Verification items for the finished model (mm, model axes). Face numbers are marked on the shaded views. A direction names the side the tool comes from. Coordinates: 2 decimals unless noted, no trailing zeros. Loops run counter-clockwise (first coordinate to the right, second up) from the corner with the lowest first, then second, coordinate; pieces in that order, holes last. Notation, with made-up numbers: (-6.5, -22.75) -> (23.5, -22.75) arc R5 ccw to (23.5, -17.75) -> close; hole circle Ø4 at (23, 5). An arc over 180 degrees is marked (long way). Answer as a JSON object with one key per item and string values. Group by question number.
Q1. Cross-section at A-A on x = 930.5. Record the boundary of the cut face in (y, z).
Q2. Cross-section at C-C on z = 60.5. Record the boundary of the cut face in (x, y).
Q3. Scan lines: L1, parallel to Z at x = 25, y = 391.1; L2, parallel to Z at x = 851, y = 26; L3, parallel to Y at x = 1153, z = 30. Record each from-to range of solid material in increasing order.
Q4. Set-up check for the marked faces 1, 2 and 3: record each of +Z, -Z, +X, -X, +Y, -Y from which the full face is reachable in a straight line by a thin tool's end or side.
Q5. Gauge pin test, flat ends, axial feed: pin 1 Ø4 at (x, z) = (692, 48) entering from -Y; pin 2 Ø4 at (x, y) = (1523, 350) entering from +Z; pin 3 Ø15.5 at (x, z) = (545, 204.8) entering from +Y; pin 4 Ø11 at (x, z) = (25, 174.8) entering from +Y. Record the tip position at first contact, or that the pin passes through.
Q6. Cross-section at B-B on y = 361.5. Record the boundary of the cut face in (x, z).
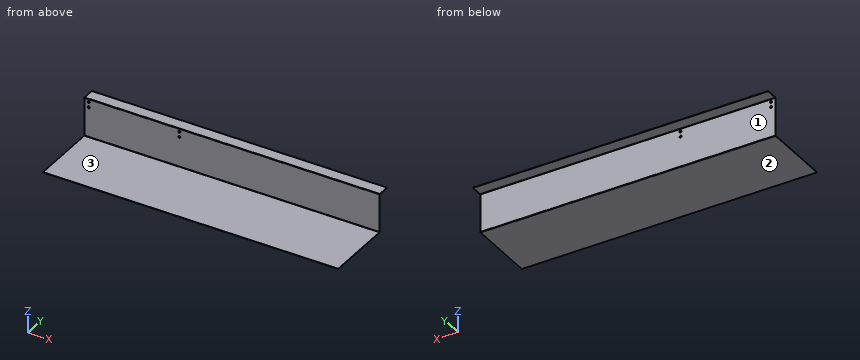
Autodesk Inventor part; units mm, degrees
ref_plane "YZ Plane" through (0, 0, 0) normal (1, 0, 0) x (0, 1, 0)
ref_plane "XZ Plane" through (0, 0, 0) normal (0, 1, 0) x (-1, 0, 0)
ref_plane "XY Plane" through (0, 0, 0) normal (0, 0, 1) x (1, 0, 0)
sketch "Sketch1" plane through (0, 0, 0) normal (0, 0, 1) x (1, 0, 0)
  line L0 (0, 0) -> (0, 392)
  line L1 (0, 392) -> (1695, 392)
  line L2 (1695, 392) -> (1695, 0)
  line L3 (1695, 0) -> (0, 0)
  dimension "d0" = 392
  dimension "d1" = 1695
extrude "Plate1" add sketch "Sketch1" along normal blind 1.6
sketch "Sketch2" plane through (1695, 390.4, 0) normal (0, 1, 0) x (-1, 0, 0)
  line L0 (1695, 0) -> (0, 0)
  line L1 (0, 0) -> (0, -223)
  line L2 (0, -223) -> (1695, -223)
  line L3 (1695, -223) -> (1695, 0)
edge flange "Flange1" height 223 angle 90 thickness 1.6 bend radius 1.6 thickness toward (0, 1, 0) relief tear relief width 1.6 relief depth 0.8 edges at (847.5, 392, 0) wall of the first edge with corners at (0, 390.4, 0) (1695, 390.4, 0) (1695, 390.4, 223) (0, 390.4, 223)
bend "Bend1"
corner "Corner1"
sketch "Sketch3" plane through (0, 390.4, 221.4) normal (0, 0, 1) x (1, 0, 0)
  line L0 (1695, 0) -> (0, 0)
  line L1 (0, 0) -> (0, -70)
  line L2 (0, -70) -> (1695, -70)
  line L3 (1695, -70) -> (1695, 0)
edge flange "Flange2" height 70 angle -90 thickness 1.6 bend radius 1.6 thickness toward (0, 0, 1) relief tear relief width 1.6 relief depth 0.8 edges at (847.5, 390.4, 223) wall of the first edge with corners at (1695, 390.4, 221.4) (0, 390.4, 221.4) (0, 460.4, 221.4) (1695, 460.4, 221.4)
bend "Bend2"
corner "Corner2"
sketch "Sketch4" plane through (0, 390.4, 3.2) normal (0, -1, 0) x (1, 0, 0)
  line L0 (0, 0) -> (0, 216.6)
  line L1 (0, 216.6) -> (0, 156.6)
  line L2 (0, 156.6) -> (1695, 156.6)
  line L3 (1695, 216.6) -> (1695, 0)
  line L4 (1695, 216.6) -> (0, 216.6)
  line L5 (1695, 156.6) -> (1695, 216.6)
  line L6 (1695, 216.6) -> (0, 216.6)
  circle A0 centre (25, 201.6) radius 6
  circle A1 centre (25, 171.6) radius 6
  circle A2 centre (545, 201.6) radius 6
  circle A3 centre (545, 171.6) radius 6
  line L7 (0, 156.6) -> (570, 156.6)
  line L8 (570, 156.6) -> (570, 216.6)
  point P0 (0, -3.2)
  dimension "d23" = 60
  dimension "d24" = 12
  dimension "d25" = 12
  dimension "d26" = 25
  dimension "d27" = 25
  dimension "d28" = 15
  dimension "d29" = 15
  dimension "d30" = 12
  dimension "d31" = 12
  dimension "d41" = 570
  dimension "d42" = 15
  dimension "d43" = 15
  dimension "d44" = 25
  dimension "d45" = 25
hole "Hole1" at (25, 390.4, 204.8) at (25, 390.4, 174.8) at (545, 390.4, 204.8) at (545, 390.4, 174.8) direction (0, 1, 0) diameter 12 end through all
equation "\"d39\" = Thickness"
equation "\"d3\" = BendReliefWidth"
equation "\"d4\" = BendReliefDepth"
equation "\"d5\" = MinimumRemnant"
equation "\"d6\" = BendRadius"
equation "\"d9\" = BendRadius"
equation "\"d10\" = CornerReliefSize"
equation "\"d11\" = GapSize"
equation "\"d12\" = JacobiRadiusSize"
equation "\"d13\" = BendReliefWidth"
equation "\"d14\" = BendReliefDepth"
equation "\"d15\" = MinimumRemnant"
equation "\"d16\" = BendRadius"
equation "\"d19\" = BendRadius"
equation "\"d20\" = CornerReliefSize"
equation "\"d21\" = GapSize"
equation "\"d22\" = JacobiRadiusSize"
equation "\"BendRadius\" = Thickness"
equation "\"BendReliefWidth\" = Thickness"
equation "\"BendReliefDepth\" = 0.5 * Thickness"
equation "\"CornerReliefSize\" = 4 * Thickness"
equation "\"MinimumRemnant\" = 2 * Thickness"
equation "\"TransitionRadius\" = BendRadius"
equation "\"JacobiRadiusSize\" = BendRadius"
equation "\"GapSize\" = Thickness"
equation "\"d2\" = BendRadius"
properties part number "MC Part4" material "Steel, Mild"
Computed values:
{
 "1": {"outline": "(0, 0) -> (388.8, 0) arc R3.2 ccw to (392, 3.2) -> (392, 219.8) arc R1.6 cw to (393.6, 221.4) -> (460.4, 221.4) -> (460.4, 223) -> (393.6, 223) arc R3.2 ccw to (390.4, 219.8) -> (390.4, 3.2) arc R1.6 cw to (388.8, 1.6) -> (0, 1.6) -> close"},
 "2": {"outline": "(0, 390.4) -> (1695, 390.4) -> (1695, 392) -> (0, 392) -> close"},
 "3": {"L1": "z = 0.98 to 168.8, 180.8 to 198.8, 210.8 to 221.8", "L2": "z = 0 to 1.6", "L3": "y = 390.4 to 392"},
 "4": {"face 1": "-Z, +X, -X, +Y", "face 2": "-Z, +X, -X, +Y, -Y", "face 3": "+Z, +X, -X, -Y"},
 "5": {"pin 1": "stops at y = 390.4", "pin 2": "stops at z = 1.6", "pin 3": "stops at y = 392", "pin 4": "passes through"},
 "6": {"outline": "(0, 0) -> (1695, 0) -> (1695, 1.6) -> (0, 1.6) -> close"}
}
